Read the model definition and answer for the solid it produces. Units are mm, in the model's axes. Face numbers are marked on the shaded views. Give positions to 0.01 mm unless a question says otherwise; leave off trailing zeros. Write each loop counter-clockwise with the first axis right and the second up, starting at its lowest first coordinate (ties: lowest second). Pieces come first, ordered by that corner, then holes.
Autodesk Inventor part; units mm, degrees
ref_plane "YZ Plane" through (0, 0, 0) normal (1, 0, 0) x (0, 1, 0)
ref_plane "XZ Plane" through (0, 0, 0) normal (0, 1, 0) x (-1, 0, 0)
ref_plane "XY Plane" through (0, 0, 0) normal (0, 0, 1) x (1, 0, 0)
sketch "Sketch_8" plane through (0, 0, 0) normal (0, 0, 1) x (1, 0, 0)
  line L0 (36, 0) -> (0, 0)
  line L1 (0, 7) -> (1, 6)
  line L2 (1, 6) -> (35, 6)
  line L3 (35, 6) -> (36, 7)
  line L4 (36, 7) -> (36, 14)
  line L5 (36, 14) -> (35, 15)
  line L6 (35, 15) -> (22, 15)
  arc A0 (20, 17) -> (22, 15) centre (22, 17) ccw
  line L7 (20, 17) -> (20, 19)
  line L8 (20, 19) -> (19, 20)
  line L9 (19, 20) -> (1, 20)
  line L10 (1, 20) -> (0, 19)
  line L11 (0, 19) -> (0, 7)
revolve "Revolution1" add sketch "Sketch_8" angle 360 about axis through (36, 0, 0) along (1, 0, 0)
properties part number "歯車m2,z18"
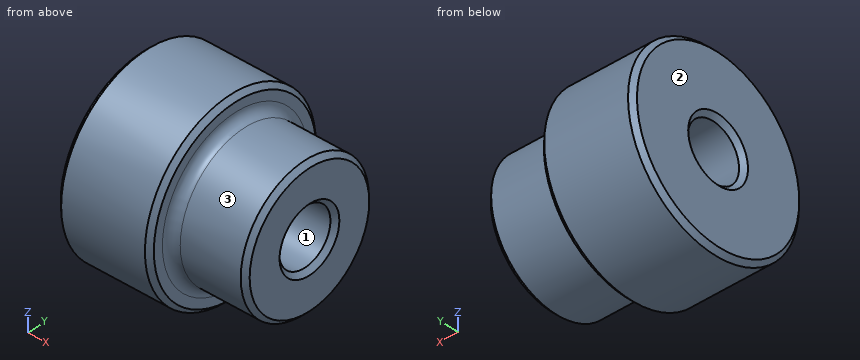
Item 1: Each of these flat-tipped pins is pushed along its axis until it touches: pin 1 Ø5 at (y, z) = (6.5, -2) entering from +X; pin 2 Ø5 at (x, z) = (28.5, -2.5) entering from -Y; pin 3 Ø10 at (x, y) = (18.5, -3) entering from +Z; pin 4 Ø5 at (x, y) = (16.5, -3) entering from -Z. Where does it stop, or does it pass through?
Result set:
pin 1: stops at x = 36
pin 2: stops at y = -15
pin 3: stops at z = 20
pin 4: stops at z = -19.99
Item 2: Section D-D (x = 26) is taken. Write down the section's boundary in (y, z), and give its area (3 significant figures).
Result set:
outline: circle Ø30 at (0, 0); hole circle Ø12 at (0, 0)
area: 594 mm2
Item 3: Determine the mould class of the marked faces 1, 2 and 3 for opening direction Y: pulls with the +Y half, pulls with the -Y half, needs draft (parallel to the pull), parting line crosses it, or undercut.
Result set:
face 1: undercut
face 2: needs draft
face 3: parting line crosses it
Item 4: Section C-C (x = 11) is taken. Write down the section's boundary in (y, z).
Result set:
outline: circle Ø40 at (0, 0); hole circle Ø12 at (0, 0)
Item 5: Find the intervals of material crossed by line 1 along Z through (x, y) = (10, 0); line 2 along Y through (x, z) = (32.5, -4.5), in increasing order.
Result set:
line 1: z = -20 to -6, 6 to 20
line 2: y = -14.31 to -3.97, 3.97 to 14.31
Item 6: Section A-A (y = 0) is taken. Write down the section's boundary in (x, z), and give its area (3 significant figures).
Result set:
outline: (0, -19) - (1, -20) - (19, -20) - (20, -19) - (20, -17) arc R2 cw to (22, -15) - (35, -15) - (36, -14) - (36, -7) - (35, -6) - (1, -6) - (0, -7) - close; (0, 7) - (1, 6) - (35, 6) - (36, 7) - (36, 14) - (35, 15) - (22, 15) arc R2 cw to (20, 17) - (20, 19) - (19, 20) - (1, 20) - (0, 19) - close
area: 845 mm2
